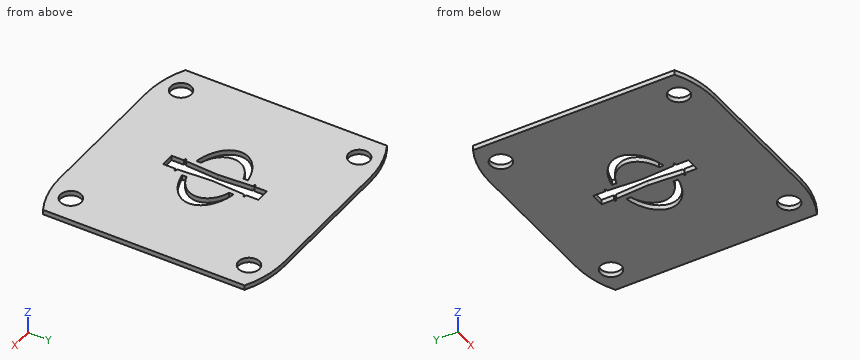
from build123d import *

# Parameters (mm, degrees)
F0_R     = 1.7272
F1_DEPTH = 0.79375
F3_DEPTH = 25.4


# Not quite as in the source:
# - a feature names something its author has since deleted; it is built from what else it names


with BuildPart() as f1:
    # F0 (on Top) → F1 (new body)
    with BuildSketch(Plane.XY):
        with BuildLine():
            Line((-19.05, 16.66875), (-19.05, 0))
            Line((-19.05, 0), (-19.05, -16.66875))
            ThreePointArc((-19.05, -16.66875), (-15.4310103444, -18.0612265152), (-11.5824, -18.5348037427))
            Line((-11.5824, -18.5348037427), (0, -18.5348037427))
            Line((0, -18.5348037427), (11.5824, -18.5348037427))
            ThreePointArc((11.5824, -18.5348037427), (15.4310103444, -18.0612265152), (19.05, -16.66875))
            Line((19.05, -16.66875), (19.05, 0))
            Line((19.05, 0), (19.05, 16.66875))
            ThreePointArc((19.05, 16.66875), (15.4310103444, 18.0612265152), (11.5824, 18.5348037427))
            Line((11.5824, 18.5348037427), (0, 18.5348037427))
            Line((0, 18.5348037427), (-11.5824, 18.5348037427))
            ThreePointArc((-11.5824, 18.5348037427), (-15.4310103444, 18.0612265152), (-19.05, 16.66875))
        make_face()
        with Locations((-14.732, -14.732)):
            Circle(F0_R, mode=Mode.SUBTRACT)
        with Locations((14.732, -14.732)):
            Circle(F0_R, mode=Mode.SUBTRACT)
        with Locations((-14.732, 14.732)):
            Circle(F0_R, mode=Mode.SUBTRACT)
        with Locations((14.732, 14.732)):
            Circle(F0_R, mode=Mode.SUBTRACT)
    extrude(amount=F1_DEPTH)

    # F2 (on face) → F3 (cut)
    with BuildSketch(Plane.XY.offset(0.79375)):
        with BuildLine():
            Line((-1.381887138, -5.588), (-1.524, -5.588))
            Line((-1.524, -5.588), (-1.524, -5.842))
            Line((-1.524, -5.842), (-1.143, -5.842))
            Line((-1.143, -5.842), (-1.143, -7.874))
            Line((-1.143, -7.874), (0, -7.874))
            Line((0, -7.874), (1.143, -7.874))
            Line((1.143, -7.874), (1.143, -5.842))
            Line((1.143, -5.842), (1.524, -5.842))
            Line((1.524, -5.842), (1.524, -5.588))
            Line((1.524, -5.588), (1.381887138, -5.588))
            ThreePointArc((1.381887138, -5.588), (1.2078708338, -5.5190252033), (1.128364287, -5.349561621))
            Line((1.128364287, -5.349561621), (0.8, 0))
            Line((0.8, 0), (1.128364287, 5.349561621))
            ThreePointArc((1.128364287, 5.349561621), (1.2078708338, 5.5190252033), (1.381887138, 5.588))
            Line((1.381887138, 5.588), (1.524, 5.588))
            Line((1.524, 5.588), (1.524, 5.842))
            Line((1.524, 5.842), (1.143, 5.842))
            Line((1.143, 5.842), (1.143, 7.874))
            Line((1.143, 7.874), (0, 7.874))
            Line((0, 7.874), (-1.143, 7.874))
            Line((-1.143, 7.874), (-1.143, 5.842))
            Line((-1.143, 5.842), (-1.524, 5.842))
            Line((-1.524, 5.842), (-1.524, 5.588))
            Line((-1.524, 5.588), (-1.381887138, 5.588))
            ThreePointArc((-1.381887138, 5.588), (-1.2078708338, 5.5190252033), (-1.128364287, 5.349561621))
            Line((-1.128364287, 5.349561621), (-0.8, 0))
            Line((-0.8, 0), (-1.128364287, -5.349561621))
            ThreePointArc((-1.128364287, -5.349561621), (-1.2078708338, -5.5190252033), (-1.381887138, -5.588))
        make_face()
        with BuildLine():
            add(Edge.make_bspline(
                [(-1.922114287, 3.5267450469), (-13.4260486871, 0), (-1.922114287, -3.5267450469)],
                knots=[1.958829942, 1.958829942, 1.958829942, 4.3243553652, 4.3243553652, 4.3243553652], degree=2, weights=[1, 0.3783689541, 1]))
            Line((-1.922114287, 3.5267450469), (-1.922114287, 4.2733939342))
            add(Edge.make_bspline(
                [(-1.922114287, 4.2733939342), (-25.3836232991, 0), (-1.922114287, -4.2733939342)],
                knots=[1.8495705702, 1.8495705702, 1.8495705702, 4.433614737, 4.433614737, 4.433614737], degree=2, weights=[1, 0.2751774212, 1]))
            Line((-1.922114287, -4.2733939342), (-1.922114287, -3.5267450469))
        make_face()
        with BuildLine():
            Line((1.922114287, 4.2733939342), (1.922114287, 3.5267450469))
            add(Edge.make_bspline(
                [(1.922114287, -3.5267450469), (13.4260486871, 0), (1.922114287, 3.5267450469)],
                knots=[5.1004225956, 5.1004225956, 5.1004225956, 7.4659480188, 7.4659480188, 7.4659480188], degree=2, weights=[1, 0.3783689541, 1]))
            Line((1.922114287, -3.5267450469), (1.922114287, -4.2733939342))
            add(Edge.make_bspline(
                [(1.922114287, -4.2733939342), (25.3836232991, 0), (1.922114287, 4.2733939342)],
                knots=[4.9911632238, 4.9911632238, 4.9911632238, 7.5752073906, 7.5752073906, 7.5752073906], degree=2, weights=[1, 0.2751774212, 1]))
        make_face()
    extrude(amount=-F3_DEPTH, mode=Mode.SUBTRACT)


solid = f1.part
Here's how the part is built. I have some questions about the finished solid (model axes, mm). Coordinates: 2 decimals unless noted, no trailing zeros. Write each loop counter-clockwise with the first axis right and the second up, starting at its lowest first coordinate (ties: lowest second). Pieces come first, ordered by that corner, then holes.
1) I'm going to push a flat-ended pin straight in: pin 1 (3 mm diameter, centred on x = 14.732, y = 14.732, fed in from +Z). Where does the tip first touch, or does it pass through?
Filled in:
pin 1: passes through
2) If we section it at A-A (y = 6.5): List the corners of the cut face in (x, z) for me.
Filled in:
outline: (-19.05, 0) - (-1.14, 0) - (-1.14, 0.79) - (-19.05, 0.79) - close; (1.14, 0) - (19.05, 0) - (19.05, 0.79) - (1.14, 0.79) - close
3) If I drill on line 1 (Y direction, x = 0.5, z = 0.7); line 2 (X direction, y = 15, z = 0.3); line 3 (Y direction, x = 3, z = 0.4), over which ranges is the centre line in solid material (lowest first)?
Filled in:
line 1: y = -18.53 to -7.87, 7.87 to 18.53
line 2: x = -19.05 to -16.44, -13.03 to 13.03, 16.44 to 19.05
line 3: y = -18.53 to -4.01, -3.07 to 3.07, 4.01 to 18.53
4) If we section it at D-D (z = 0.3): Count the separate pieces of the cut face and the enclosed holes in it, plus the area to 3 significant figures.
Filled in:
separate pieces: 1
enclosed holes: 7
area: 1,290 mm2
5) If we section it at B-B (x = -15): List the corners of the cut face in (y, z) for me, plus the area to 3 significant figures.
Filled in:
outline: (-18.16, 0) - (-16.44, 0) - (-16.44, 0.79) - (-18.16, 0.79) - close; (-13.03, 0) - (13.03, 0) - (13.03, 0.79) - (-13.03, 0.79) - close; (16.44, 0) - (18.16, 0) - (18.16, 0.79) - (16.44, 0.79) - close
area: 23.4 mm2
6) If we section it at C-C (y = 14): List the corners of the cut face in (x, z) for me.
Filled in:
outline: (-19.05, 0) - (-16.3, 0) - (-16.3, 0.79) - (-19.05, 0.79) - close; (-13.17, 0) - (13.17, 0) - (13.17, 0.79) - (-13.17, 0.79) - close; (16.3, 0) - (19.05, 0) - (19.05, 0.79) - (16.3, 0.79) - close
